Part model, mm, in its own coordinate system. Face numbers are marked on the shaded views. A direction names the side the tool comes from. Coordinates: 2 decimals unless noted, no trailing zeros. One line per question, with ' | ' between items. Start each with the question number.
Item 1: Probe probe 1 along X at (y, z) = (-31.75, -12.5); probe 2 along Z at (x, y) = (-3, -34); probe 3 along Y at (x, z) = (-24.5, -5.25). List the from-to ranges inside material, lowest first. Write a range as [from, to].
Item 2: Pin check, flat tips, straight feed: pin 1 (1.7 mm diameter, centred on x = -23.5, y = -32, fed in from -Z); pin 2 (1.4 mm diameter, centred on x = -23.83, y = -31.75, fed in from -Z). Stop position of each tip, or through.
Item 3: 3-axis set-ups, long thin cutter, end or side, ignore diameter. For the marked faces 5 and 6: which of +Z, -Z, +X, -X, +Y, -Y reach the whole face in a straight line?
Item 4: Two-plate mould, pull along X, no slides. Class the marked faces 1, 2, 3 and 4: pulls with the +X half, pulls with the -X half, needs draft (parallel to the pull), parting line crosses it, or undercut.
from build123d import *

# Parameters (mm, degrees)
F0_W     = 60.325
F0_H     = 26.9875
F1_DEPTH = 57.15
F2_R     = 1.5875
F3_R     = 0.79375
F4_DEPTH = 12.7


with BuildPart() as f1:
    # F0 (on Front) → F1 (new body)
    with BuildSketch(Plane.XZ):
        with Locations((0, -2.493597)):
            Rectangle(F0_W, F0_H)
        Polygon((-6.35, 5.106403), (6.35, 5.106403), (6.35, -2.493597), (3.65, -2.493597), (3.65, -4.293597), (2.55, -4.293597), (2.55, -5.593597), (-2.55, -5.593597), (-2.55, -4.293597), (-3.65, -4.293597), (-3.65, -2.493597), (-6.35, -2.493597), align=None, mode=Mode.SUBTRACT)
    extrude(amount=F1_DEPTH)

    # F2
    f2_edges = [f1.edges().sort_by_distance(p)[0] for p in [
        (-30.1625, -28.575, 11.000153),
        (0, -57.15, 11.000153),
        (-30.1625, -57.15, -2.493597),
        (-30.1625, 0, -2.493597),
        (0, 0, 11.000153),
        (30.1625, -28.575, 11.000153),
        (30.1625, 0, -2.493597),
        (30.1625, -57.15, -2.493597),
    ]]
    fillet(f2_edges, radius=F2_R)

    # F3 (on face) → F4 (cut)
    with BuildSketch(Plane(origin=(0, 0, -15.987347), x_dir=(1, 0, 0), z_dir=(0, 0, -1))):
        with Locations((23.8252, 31.75)):
            Circle(F3_R)
        with Locations((-23.8252, 31.75)):
            Circle(F3_R)
    extrude(amount=-F4_DEPTH, mode=Mode.SUBTRACT)


solid = f1.part
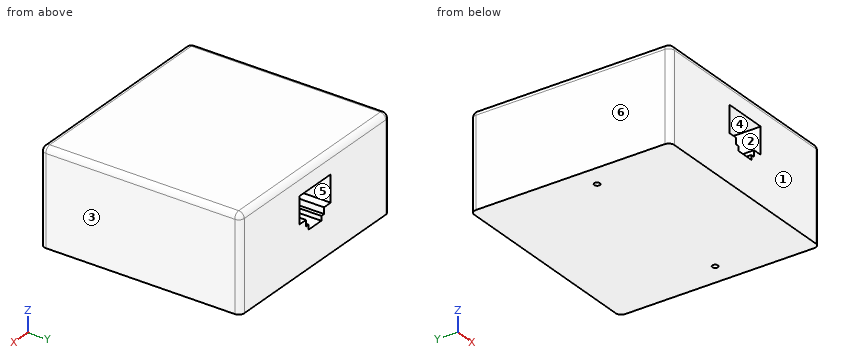
From the geometry:
1) probe 1: [-30.16, -24.62], [-23.03, 23.03], [24.62, 30.16] | probe 2: [-15.99, -4.29], [5.11, 11] | probe 3: [-57.15, -32.17], [-31.33, 0]
2) pin 1: z = -15.99 | pin 2: z = -3.29
3) face 5: +Y, -Y | face 6: +Z, -Z, -X, +Y, -Y
4) face 1: needs draft | face 2: undercut | face 3: pulls with the +X half | face 4: undercut
